Can you work these out from the model? Positions are in its coordinate system, mm. Face numbers are marked on the shaded views. A direction names the side the tool comes from. Coordinates: 2 decimals unless noted, no trailing zeros. Order: outer loops, then holes, each group sorted by start corner. A loop starts at its lowest first (then second) coordinate and runs counter-clockwise, first axis right, second up. Notation, with made-up numbers: (21, -2) -> (37, -2) arc R28 cw to (37, 19) -> close; hole circle Ø1 at (-30.75, -26). An arc over 180 degrees is marked (long way). Use a Markdown table: item, result. Add a question column.
1. If I drill on line 1 along Y through (x, z) = (158.25, 2.3); line 2 along Y through (x, z) = (151, 2.95); line 3 along X through (y, z) = (206, 1.55), over which ranges is the centre line in solid material (lowest first)? Write a range as from..to.
2. Suppose I cut it at C-C, the plane z = 2.35. List the corners of the cut face in (x, y) for me, then the cut area to 3 significant figures.
3. For the marked faces 1, 2 and 3, which set-ups out of +Z, -Z, +X, -X, +Y, -Y let a thin tool reach every point of the face, with its end or its side?
4. Suppose I cut it at D-D, the plane x = 159.5. List the corners of the cut face in (y, z) for me.
5. Suppose I cut it at B-B, the plane x = 151. List the corners of the cut face in (y, z) for me.
6. Suppose I cut it at A-A, the plane y = 199.25. List the corners of the cut face in (x, z) for me, then the cut area to 4 significant figures.
7. We'd pull the mould along Y, two halves only. Please class the marked faces 4, 5 and 6: pulls with the +Y half, pulls with the -Y half, needs draft (parallel to the pull), parting line crosses it, or undercut.
8. For pin 1 Ø0.5 at (x, z) = (158.5, 2) entering from -Y; pin 2 Ø1.5 at (x, z) = (148, 1.5) entering from +Y; pin 3 Ø0.9 at (y, z) = (198.5, 1) entering from -X, each with a flat end and sliding along its axis, tell me the tip position at first contact or that it passes through.
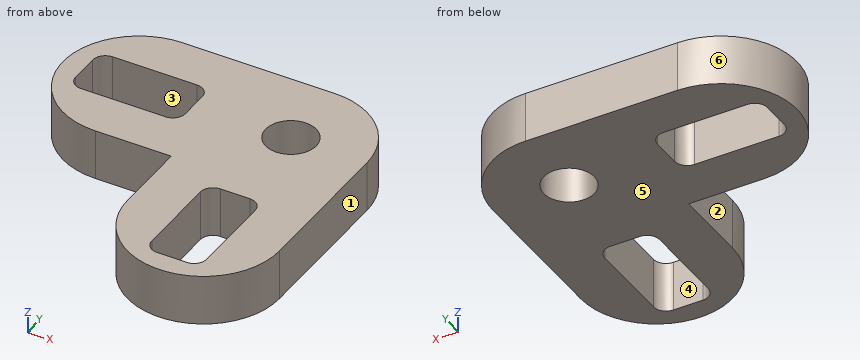
```python
from build123d import *

# Parameters (mm, degrees)
MODEL_R                 = 1.5
SALIENTE_EXTRUIR1_DEPTH = 3


with BuildPart() as part:
    # Model → Saliente-Extruir1 (new body)
    with BuildSketch(Plane.XY):
        with BuildLine():
            Line((149.34213351, 211.823953209), (158.34213351, 211.823953209))
            ThreePointArc((158.34213351, 211.823953209), (161.524114025, 210.505933724), (162.84213351, 207.323953209))
            Line((162.84213351, 207.323953209), (162.84213351, 198.323953209))
            ThreePointArc((162.84213351, 198.323953209), (158.34213351, 193.823953209), (153.84213351, 198.323953209))
            Line((153.84213351, 198.323953209), (153.84213351, 202.823953209))
            Line((153.84213351, 202.823953209), (149.34213351, 202.823953209))
            ThreePointArc((149.34213351, 202.823953209), (144.84213351, 207.323953209), (149.34213351, 211.823953209))
        make_face()
        with Locations((158.34213351, 207.323953209)):
            Circle(MODEL_R, mode=Mode.SUBTRACT)
        with BuildLine():
            Line((156.71713351, 195.823953209), (156.71713351, 200.823953209))
            ThreePointArc((156.71713351, 200.823953209), (156.936803424, 201.354283295), (157.46713351, 201.573953209))
            Line((157.46713351, 201.573953209), (159.21713351, 201.573953209))
            ThreePointArc((159.21713351, 201.573953209), (159.747463595, 201.354283295), (159.96713351, 200.823953209))
            Line((159.96713351, 200.823953209), (159.96713351, 195.823953209))
            ThreePointArc((159.96713351, 195.823953209), (159.747463595, 195.293623123), (159.21713351, 195.073953209))
            Line((159.21713351, 195.073953209), (157.46713351, 195.073953209))
            ThreePointArc((157.46713351, 195.073953209), (156.936803424, 195.293623123), (156.71713351, 195.823953209))
        make_face(mode=Mode.SUBTRACT)
        with BuildLine():
            Line((151.84213351, 205.698953209), (146.84213351, 205.698953209))
            ThreePointArc((146.84213351, 205.698953209), (146.311803424, 205.918623123), (146.09213351, 206.448953209))
            Line((146.09213351, 206.448953209), (146.09213351, 208.198953209))
            ThreePointArc((146.09213351, 208.198953209), (146.311803424, 208.729283295), (146.84213351, 208.948953209))
            Line((146.84213351, 208.948953209), (151.84213351, 208.948953209))
            ThreePointArc((151.84213351, 208.948953209), (152.372463595, 208.729283295), (152.59213351, 208.198953209))
            Line((152.59213351, 208.198953209), (152.59213351, 206.448953209))
            ThreePointArc((152.59213351, 206.448953209), (152.372463595, 205.918623123), (151.84213351, 205.698953209))
        make_face(mode=Mode.SUBTRACT)
    extrude(amount=SALIENTE_EXTRUIR1_DEPTH)


solid = part.part
```
Worked out:
| question | item | result |
|---|---|---|
| 1 | line 1 | y = 193.82..195.07, 201.57..205.83, 208.82..211.82 |
| 1 | line 2 | y = 202.82..205.7, 208.95..211.82 |
| 1 | line 3 | x = 145.04..146.24, 152.44..157.64, 159.05..162.84 |
| 2 | outline | (149.34, 202.82) -> (153.84, 202.82) -> (153.84, 198.32) arc R4.5 ccw to (162.84, 198.32) -> (162.84, 207.32) arc R4.5 ccw to (158.34, 211.82) -> (149.34, 211.82) arc R4.5 ccw to start; hole (146.09, 206.45) arc R0.75 ccw to (146.84, 205.7) -> (151.84, 205.7) arc R0.75 ccw to (152.59, 206.45) -> (152.59, 208.2) arc R0.75 ccw to (151.84, 208.95) -> (146.84, 208.95) arc R0.75 ccw to (146.09, 208.2) -> close; hole (156.72, 195.82) arc R0.75 ccw to (157.47, 195.07) -> (159.22, 195.07) arc R0.75 ccw to (159.97, 195.82) -> (159.97, 200.82) arc R0.75 ccw to (159.22, 201.57) -> (157.47, 201.57) arc R0.75 ccw to (156.72, 200.82) -> close; hole circle Ø3 at (158.34, 207.32) |
| 2 | area | 173 mm² |
| 3 | face 1 | +Z, -Z, +X, +Y, -Y |
| 3 | face 2 | +Z, -Z, -X, -Y |
| 3 | face 3 | +Z, -Z |
| 4 | outline | (193.98, 0) -> (195.13, 0) -> (195.13, 3) -> (193.98, 3) -> close; (201.52, 0) -> (206.37, 0) -> (206.37, 3) -> (201.52, 3) -> close; (208.28, 0) -> (211.67, 0) -> (211.67, 3) -> (208.28, 3) -> close |
| 5 | outline | (202.82, 0) -> (205.7, 0) -> (205.7, 3) -> (202.82, 3) -> close; (208.95, 0) -> (211.82, 0) -> (211.82, 3) -> (208.95, 3) -> close |
| 6 | outline | (153.84, 0) -> (156.72, 0) -> (156.72, 3) -> (153.84, 3) -> close; (159.97, 0) -> (162.84, 0) -> (162.84, 3) -> (159.97, 3) -> close |
| 6 | area | 17.25 mm² |
| 7 | face 4 | undercut |
| 7 | face 5 | needs draft |
| 7 | face 6 | parting line crosses it |
| 8 | pin 1 | stops at y = 193.82 |
| 8 | pin 2 | stops at y = 211.78 |
| 8 | pin 3 | stops at x = 153.84 |
